Check sheet for the modelled part. Datum: model origin and axes. Units: mm. Face numbers are marked on the shaded views. A direction names the side the tool comes from. Coordinates: 2 decimals unless noted, no trailing zeros. Loops run counter-clockwise (first coordinate to the right, second up) from the corner with the lowest first, then second, coordinate; pieces in that order, holes last. Notation, with made-up numbers: (18, 54) - (71, 54) arc R17 cw to (71, 62) - close; hole circle Ø9 at (72.25, 77.25). An arc over 180 degrees is marked (long way). Write each question's results on one line, items separated by ' | '. Start each with the question number.
1. Tool access check on the marked faces 3 and 4. Record the directions out of +Z, -Z, +X, -X, +Y, -Y that give a thin tool (end or side, any length) a straight path to the whole face; none if there is none.
2. Thickness scan on line 1 (Z direction, x = -267, y = 67); line 2 (Z direction, x = -263.5, y = 65); line 3 (X direction, y = 106, z = 54). Record the ranges inside material, lowest first. Write a range as [from, to].
3. Cross-section at A-A (z = 45). Record the cut outline in (x, y).
4. Gauge pin test, flat ends, axial feed: P1, Ø3, axis at y = 78.5, z = 29, coming from the +X side; P2, Ø12, axis at x = -264.5, y = 87.5, coming from the +Z side; P3, Ø16, axis at x = -251.15, z = 48.95, coming from the +Y side. Record the tip position at first contact, or that the pin passes through.
5. Cross-section at C-C (z = 23). Record the cut outline in (x, y).
6. Cross-section at D-D (y = 85). Record the cut outline in (x, z).
7. Cross-section at B-B (y = 111). Record the cut outline in (x, z), and give its area (3 significant figures).
8. Draft check along Y on the marked faces 1 and 2. Enter one of: released by +Y, released by -Y, zero draft, split by the parting line, or undercut.
```python
from build123d import *

# Parameters (mm, degrees)
SPUR_START             = -273.054421635
SPUR_GEAR_AM_OUTLINE_R = 9.525
SPUR_GEAR_AM_DEPTH     = 12.7
SCALE2_SCALE           = 0.7
SKETCH5_R              = 10
CUT_EXTRUDE2_DEPTH     = 141.883332495
BOSS_EXTRUDE1_START    = 20
SKETCH7_R              = 13
SKETCH7_R_2            = 10
BOSS_EXTRUDE1_DEPTH    = 20
SKETCH8_R              = 5
CUT_EXTRUDE3_DEPTH     = 306.435901832


# Read off the part's stored shape, not the designer's step: spur gear_am
with BuildPart() as part:
    # spur gear_am outline → spur gear_am (new body)
    with BuildSketch(Plane.YZ.offset(SPUR_START)):
        with BuildLine():
            ThreePointArc((116.546862005, 16.732254346), (117.355063047, 17.520188248), (118.142996949, 18.32838929))
            ThreePointArc((118.142996949, 18.32838929), (115.759708054, 25.667921311), (110.086646287, 30.899093879))
            ThreePointArc((110.086646287, 30.899093879), (112.044558013, 33.870469671), (113.638889071, 37.05175886))
            ThreePointArc((113.638889071, 37.05175886), (121.00574829, 34.754329537), (128.553613919, 36.360106821))
            ThreePointArc((128.553613919, 36.360106821), (128.859569602, 37.446578117), (129.137839856, 38.540467701))
            ThreePointArc((129.137839856, 38.540467701), (123.404085119, 43.705044437), (115.875483227, 45.398841888))
            ThreePointArc((115.875483227, 45.398841888), (116.085396623, 48.951084671), (115.875483227, 52.503327455))
            ThreePointArc((115.875483227, 52.503327455), (123.404085118, 54.197124907), (129.137839856, 59.361701642))
            ThreePointArc((129.137839856, 59.361701642), (128.859569602, 60.455591227), (128.553613919, 61.542062523))
            ThreePointArc((128.553613919, 61.542062523), (121.00574829, 63.147839807), (113.638889071, 60.850410483))
            ThreePointArc((113.638889071, 60.850410483), (112.044558013, 64.031699672), (110.086646287, 67.003075464))
            ThreePointArc((110.086646287, 67.003075464), (115.759708054, 72.234248032), (118.142996949, 79.573780054))
            ThreePointArc((118.142996949, 79.573780054), (117.355063047, 80.381981095), (116.546862005, 81.169914997))
            ThreePointArc((116.546862005, 81.169914997), (109.207329984, 78.786626103), (103.976157416, 73.113564336))
            ThreePointArc((103.976157416, 73.113564336), (101.004781623, 75.071476061), (97.823492434, 76.665807119))
            ThreePointArc((97.823492434, 76.665807119), (100.120921758, 84.032666338), (98.515144474, 91.580531968))
            ThreePointArc((98.515144474, 91.580531968), (97.428673178, 91.88648765), (96.334783594, 92.164757905))
            ThreePointArc((96.334783594, 92.164757905), (91.170206858, 86.431003167), (89.476409406, 78.902401276))
            ThreePointArc((89.476409406, 78.902401276), (85.924166623, 79.112314672), (82.37192384, 78.902401276))
            ThreePointArc((82.37192384, 78.902401276), (80.678126388, 86.431003167), (75.513549653, 92.164757905))
            ThreePointArc((75.513549653, 92.164757905), (74.419660069, 91.88648765), (73.333188772, 91.580531968))
            ThreePointArc((73.333188772, 91.580531968), (71.727411488, 84.032666338), (74.024840812, 76.665807119))
            ThreePointArc((74.024840812, 76.665807119), (70.843551623, 75.071476061), (67.87217583, 73.113564336))
            ThreePointArc((67.87217583, 73.113564336), (62.641003263, 78.786626103), (55.301471241, 81.169914997))
            ThreePointArc((55.301471241, 81.169914997), (54.493270199, 80.381981096), (53.705336298, 79.573780054))
            ThreePointArc((53.705336298, 79.573780054), (56.088625192, 72.234248032), (61.761686959, 67.003075464))
            ThreePointArc((61.761686959, 67.003075464), (59.803775234, 64.031699671), (58.209444175, 60.850410483))
            ThreePointArc((58.209444175, 60.850410483), (50.842584956, 63.147839807), (43.294719327, 61.542062523))
            ThreePointArc((43.294719327, 61.542062523), (42.988763645, 60.455591226), (42.71049339, 59.361701642))
            ThreePointArc((42.71049339, 59.361701642), (48.444248128, 54.197124907), (55.972850019, 52.503327455))
            ThreePointArc((55.972850019, 52.503327455), (55.762936623, 48.951084671), (55.972850019, 45.398841888))
            ThreePointArc((55.972850019, 45.398841888), (48.444248127, 43.705044437), (42.71049339, 38.540467701))
            ThreePointArc((42.71049339, 38.540467701), (42.988763645, 37.446578117), (43.294719327, 36.360106821))
            ThreePointArc((43.294719327, 36.360106821), (50.842584956, 34.754329537), (58.209444175, 37.05175886))
            ThreePointArc((58.209444175, 37.05175886), (59.803775234, 33.870469672), (61.761686959, 30.899093879))
            ThreePointArc((61.761686959, 30.899093879), (56.088625192, 25.667921311), (53.705336298, 18.32838929))
            ThreePointArc((53.705336298, 18.32838929), (54.493270199, 17.520188248), (55.301471241, 16.732254346))
            ThreePointArc((55.301471241, 16.732254346), (62.641003263, 19.11554324), (67.87217583, 24.788605007))
            ThreePointArc((67.87217583, 24.788605007), (70.843551623, 22.830693282), (74.024840812, 21.236362224))
            ThreePointArc((74.024840812, 21.236362224), (71.727411488, 13.869503005), (73.333188772, 6.321637376))
            ThreePointArc((73.333188772, 6.321637376), (74.419660068, 6.015681693), (75.513549653, 5.737411439))
            ThreePointArc((75.513549653, 5.737411439), (80.678126388, 11.471166177), (82.37192384, 18.999768068))
            ThreePointArc((82.37192384, 18.999768068), (85.924166623, 18.789854672), (89.476409406, 18.999768068))
            ThreePointArc((89.476409406, 18.999768068), (91.170206858, 11.471166176), (96.334783594, 5.737411439))
            ThreePointArc((96.334783594, 5.737411439), (97.428673178, 6.015681693), (98.515144474, 6.321637376))
            ThreePointArc((98.515144474, 6.321637376), (100.120921758, 13.869503005), (97.823492434, 21.236362224))
            ThreePointArc((97.823492434, 21.236362224), (101.004781623, 22.830693282), (103.976157416, 24.788605007))
            ThreePointArc((103.976157416, 24.788605007), (109.207329984, 19.11554324), (116.546862005, 16.732254346))
        make_face()
        with Locations((85.924166623, 48.951084672)):
            Circle(SPUR_GEAR_AM_OUTLINE_R, mode=Mode.SUBTRACT)
    extrude(amount=SPUR_GEAR_AM_DEPTH)


with BuildPart() as part_1:
    # Scale2: scaled about (-266.704421635, 85.924166623, 48.951084672)
    add(part.part.scale(SCALE2_SCALE).moved(Location((-80.011326491, 25.777249987, 14.685325402))))

    # Sketch5 → Cut-Extrude2 (cut, through all)
    with BuildSketch(Plane(origin=(-262.259421635, 0, 0), x_dir=(0, 0, -1), z_dir=(1, 0, 0))):
        with Locations((-48.951084672, 85.924166623)):
            Circle(SKETCH5_R)
    extrude(amount=-CUT_EXTRUDE2_DEPTH, mode=Mode.SUBTRACT)

    # Sketch7 → Boss-Extrude1 (add)
    with BuildSketch(Plane(origin=(-262.259421635, 0, 0), x_dir=(0, 0, -1), z_dir=(1, 0, 0)).offset(BOSS_EXTRUDE1_START)):
        with Locations(Location((-48.951084672, 85.924166623, 0), (0, 0, 180))):
            Circle(SKETCH7_R)
        with Locations((-48.951084672, 85.924166623)):
            Circle(SKETCH7_R_2, mode=Mode.SUBTRACT)
    extrude(amount=-BOSS_EXTRUDE1_DEPTH)

    # Sketch8 → Cut-Extrude3 (cut, through all)
    with BuildSketch(Plane(origin=(0, 0, 0), x_dir=(1, 0, 0), z_dir=(0, 1, 0))):
        with Locations(Location((-251.149421635, -48.951084672, 0), (0, 0, 90))):
            Circle(SKETCH8_R)
    extrude(amount=CUT_EXTRUDE3_DEPTH, mode=Mode.SUBTRACT)


solid = part_1.part
```
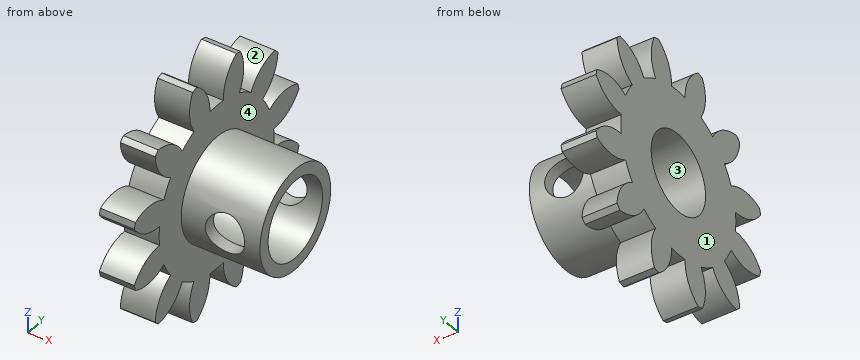
Established:
1) face 3: +X, -X | face 4: +X
2) line 1: [26.85, 34.93], [39.59, 58.31], [62.97, 71.05] | line 2: [26.44, 32.59], [39.83, 58.07], [65.31, 71.46] | line 3: [-271.15, -262.26]
3) outline: (-271.15, 59.18) - (-262.26, 59.18) - (-262.26, 73.54) - (-254.21, 73.54) - (-254.21, 76.74) - (-271.15, 76.74) - close; (-271.15, 95.11) - (-254.21, 95.11) - (-254.21, 98.31) - (-262.26, 98.31) - (-262.26, 112.67) - (-271.15, 112.67) - close; (-248.09, 73.54) - (-242.26, 73.54) - (-242.26, 76.74) - (-248.09, 76.74) - close; (-248.09, 95.11) - (-242.26, 95.11) - (-242.26, 98.31) - (-248.09, 98.31) - close
4) P1: x = -262.26 | P2: z = 79.2 | P3: y = 98.92
5) outline: (-271.15, 76.01) - (-262.26, 76.01) - (-262.26, 82.39) - (-271.15, 82.39) - close; (-271.15, 89.45) - (-262.26, 89.45) - (-262.26, 95.84) - (-271.15, 95.84) - close
6) outline: (-271.15, 27.86) - (-262.26, 27.86) - (-262.26, 35.98) - (-242.26, 35.98) - (-242.26, 38.99) - (-271.15, 38.99) - close; (-271.15, 58.91) - (-242.26, 58.91) - (-242.26, 61.92) - (-262.26, 61.92) - (-262.26, 70.04) - (-271.15, 70.04) - close
7) outline: (-271.15, 39) - (-262.26, 39) - (-262.26, 45.79) - (-271.15, 45.79) - close; (-271.15, 52.11) - (-262.26, 52.11) - (-262.26, 58.9) - (-271.15, 58.9) - close | area: 121 mm^2
8) face 1: zero draft | face 2: undercut
